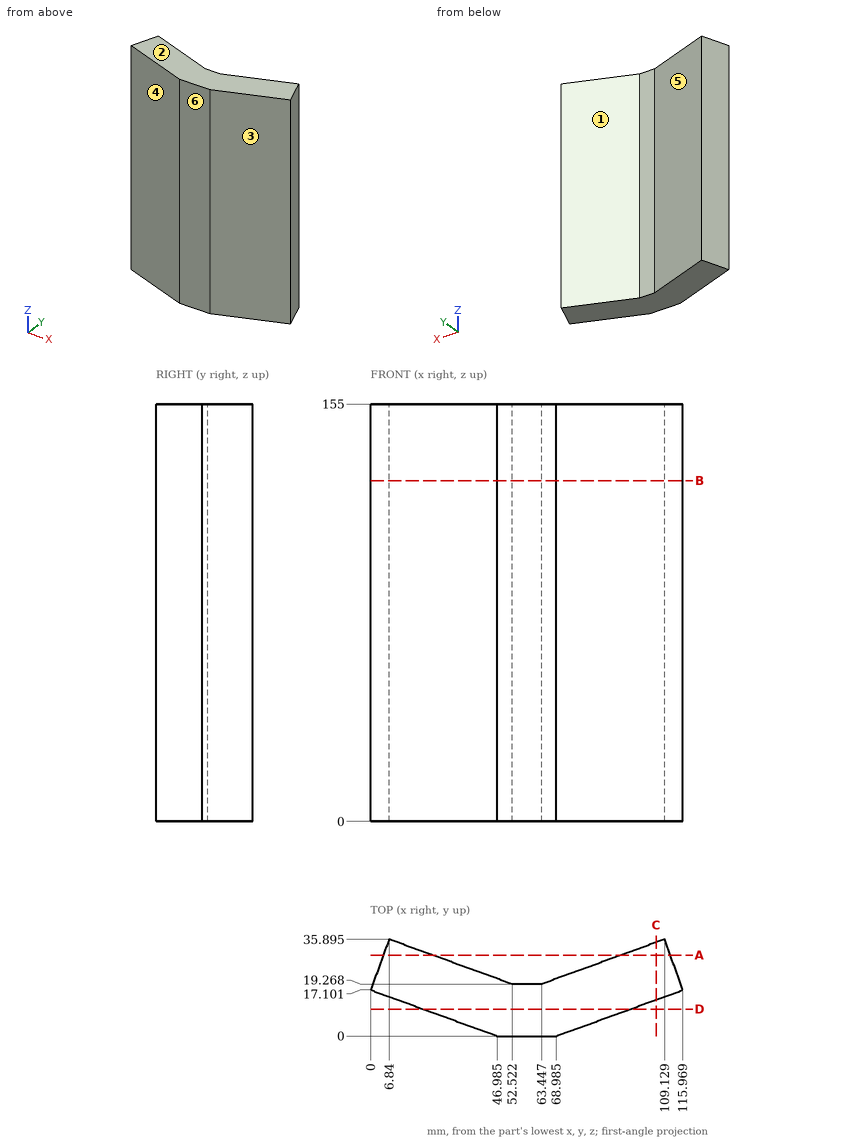
For this review, use the dimensioned drawing (mm, ordinates from the lowest corner) and the shaded views. A direction names the side the tool comes from. Coordinates: 2 decimals unless noted, no trailing zeros. Loops run counter-clockwise (first coordinate to the right, second up) from the corner with the lowest first, then second, coordinate; pieces in that order, holes last. Notation, with made-up numbers: (-15.75, 15.25) -> (-8.75, 15.25) arc R16 ccw to (-8.75, 19.25) -> close; hole circle Ø1 at (23.5, 86). An arc over 180 degrees is marked (long way). Use a Markdown table: item, result. Add a question column.
Item 1: We need section D-D, the plane y = 10. Write out the cut boundary in (x, z).
Item 2: Wall thickness on L1, parallel to Y at x = 81, z = 46; L2, parallel to Y at x = 64.5, z = 105: over which ranges is each line inside the solid? List them lowest first. Write a range as from..to.
Item 3: We need section B-B, the plane z = 126.5. Write out the cut boundary in (x, y) (1 decimal).
Item 4: The part is to be moulded in two halves that separate along X. For the marked faces 3, 4, 5 and 6, say which applies: +X half, -X half, draft (parallel to the pull), parting line (faces both ways), or undercut.
Item 5: We need section C-C, the plane x = 106. Write out the cut boundary in (y, z), and give its area (3 significant figures).
Item 6: Machinability: for the marked faces 1 and 2, which of the approach directions +Z, -Z, +X, -X, +Y, -Y give a long, thin tool a straight path to every point of the face, cutting with its end or side? Answer none if there is none.
Item 7: Clearance check with flat-ended pins moving along their axes: P1, Ø4, axis at y = 30, z = 132, coming from the -X side; P2, Ø8.5, axis at x = 56.5, z = 92.5, coming from the +Y side; P3, Ø4, axis at y = 20.5, z = 71, coming from the -X side. State where each tip first meets the part, or that it passes through.
Item 8: We need section A-A, the plane y = 30. Write out the cut boundary in (x, z) (1 decimal).
Numbers:
| question | item | result |
|---|---|---|
| 1 | outline | (19.51, 0) -> (96.46, 0) -> (96.46, 155) -> (19.51, 155) -> close |
| 2 | L1 | y = 4.37..25.66 |
| 2 | L2 | y = 0..19.65 |
| 3 | outline | (0, 17.1) -> (47, 0) -> (69, 0) -> (116, 17.1) -> (109.1, 35.9) -> (63.4, 19.3) -> (52.5, 19.3) -> (6.8, 35.9) -> close |
| 4 | face 3 | +X half |
| 4 | face 4 | -X half |
| 4 | face 5 | undercut |
| 4 | face 6 | draft |
| 5 | outline | (13.47, 0) -> (34.76, 0) -> (34.76, 155) -> (13.47, 155) -> close |
| 5 | area | 3,300 mm^2 |
| 6 | face 1 | +Z, -Z, +Y |
| 6 | face 2 | +Z, +X, -X, +Y, -Y |
| 7 | P1 | stops at x = 3.97 |
| 7 | P2 | stops at y = 19.37 |
| 7 | P3 | stops at x = 0.51 |
| 8 | outline | (4.7, 0) -> (23, 0) -> (23, 155) -> (4.7, 155) -> close; (92.9, 0) -> (111.3, 0) -> (111.3, 155) -> (92.9, 155) -> close |
